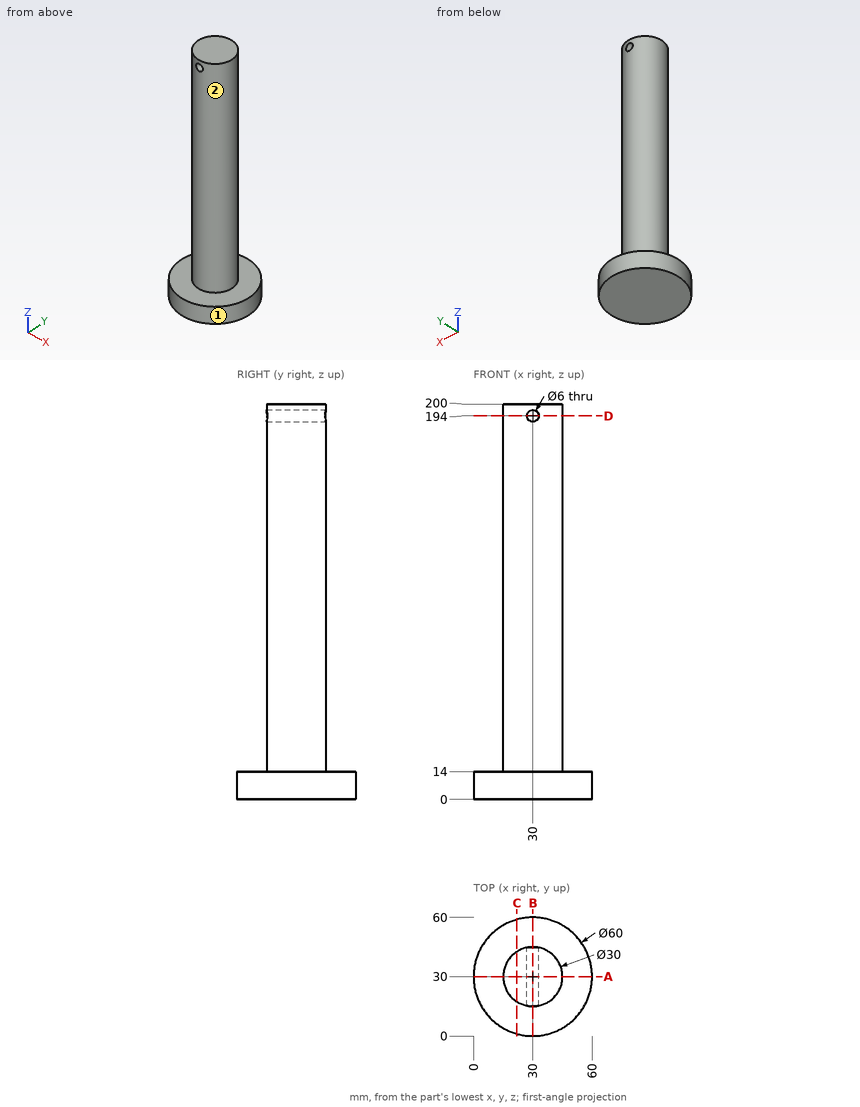
The figure shows three views and two pictorial views of one solid part (mm, origin at its lowest corner). Answer the questions. A direction names the side the tool comes from. Give positions to 0.01 mm unless a question says otherwise; leave off trailing zeros. Loops run counter-clockwise (first coordinate to the right, second up) from the corner with the lowest first, then second, coordinate; pieces in that order, holes last. Notation, with made-up numbers: (-14, 79.25) - (-5, 79.25) arc R12 ccw to (-5, 90.25) - close; hole circle Ø1 at (29, -34.75). An arc over 180 degrees is marked (long way). Use one line per item in the form item = value.
1. Which of the six approach directions +Z, -Z, +X, -X, +Y, -Y give full straight-line access (tool end or side, diameter ignored) to the marked faces 1 and 2?
Calculated:
face_1 = +Z, -Z
face_2 = +Z
2. Section D-D on z = 194 is taken. Give the vertices of the cut face in (x, y), then the cut area to 3 significant figures.
Calculated:
outline = (27, 15.3) - (27, 44.7) arc R15 ccw to start; (33, 15.3) arc R15 ccw to (33, 44.7) - close
area = 528 mm^2
3. Section B-B on x = 30 is taken. Give the vertices of the cut face in (y, z), then the cut area to 3 significant figures.
Calculated:
outline = (0, 0) - (60, 0) - (60, 14) - (45, 14) - (45, 191) - (15, 191) - (15, 14) - (0, 14) - close; (15, 197) - (45, 197) - (45, 200) - (15, 200) - close
area = 6,240 mm^2
4. Given pin 1 Ø12 at (y, z) = (26.5, 101.5) entering from -X; pin 2 Ø5 at (x, z) = (22, 38.5) entering from +Y; pin 3 Ø9.5 at (x, z) = (30, 194) entering from +Y; pin 4 Ø8 at (x, z) = (50, 48.5) entering from +Y, each flat-ended and moving along its own axis, determine where each tip first touches the part or whether it passes through.
Calculated:
pin_1 = 15
pin_2 = 43.96
pin_3 = 45
pin_4 = through
5. Section C-C on x = 22 is taken. Give the vertices of the cut face in (y, z), then the cut area to 3 significant figures.
Calculated:
outline = (1.09, 0) - (58.91, 0) - (58.91, 14) - (42.69, 14) - (42.69, 200) - (17.31, 200) - (17.31, 14) - (1.09, 14) - close
area = 5,530 mm^2
6. Section A-A on y = 30 is taken. Give the vertices of the cut face in (x, z).
Calculated:
outline = (0, 0) - (60, 0) - (60, 14) - (45, 14) - (45, 200) - (15, 200) - (15, 14) - (0, 14) - close; hole circle Ø6 at (30, 194)
7. Find the intervals of material crossed by line 1 along Z through (x, y) = (30, 28.5); line 2 along Z through (x, y) = (51, 37); line 3 along X through (y, z) = (31, 194), in increasing order. Write a range as [from, to].
Calculated:
line_1 = [0, 191], [197, 200]
line_2 = [0, 14]
line_3 = [15.03, 27], [33, 44.97]
